from build123d import *

# Parameters (mm, degrees)
EXTRUDE_1_DEPTH           = 15.5
HOLE_WIZARD_M121_D        = 10.2
HOLE_WIZARD_M121_DEPTH    = 15.5
HOLE_WIZARD_M82_D         = 6.8
HOLE_WIZARD_M82_DEPTH     = 15.5
HOLE_WIZARD_8_0_8_1_D     = 8
HOLE_WIZARD_8_0_8_1_DEPTH = 15.5
SKETCH_9_W                = 8
SKETCH_9_H                = 8
SKETCH_9_H_2              = 5
SKETCH_9_W_2              = 5
EXTRUDE_2_DEPTH           = 2
FILLET_1_R                = 2


with BuildPart() as part:
    # Эскиз1 → Бобышка-Вытянуть1 (new body)
    with BuildSketch(Plane(origin=(0, 0, 0), x_dir=(1, 0, 0), z_dir=(0, 1, 0))):
        Polygon((0, 0), (0, 120), (60, 120), (120, 60), (120, 0), align=None)
    extrude(amount=EXTRUDE_1_DEPTH)

    # Отверстие обработанное метчиком M121
    with Locations(Plane(origin=(0, 15.5, 0), x_dir=(1, 0, 0), z_dir=(0, 1, 0))):
        with Locations((60, 60)):
            Hole(HOLE_WIZARD_M121_D / 2, depth=HOLE_WIZARD_M121_DEPTH)

    # Отверстие обработанное метчиком M82
    with Locations(Plane(origin=(0, 15.5, 0), x_dir=(1, 0, 0), z_dir=(0, 1, 0))):
        with Locations((58.180194847, 107.67766953), (107.67766953, 58.180194847), (58.180194847, 8.682720164), (8.682720164, 58.180194847)):
            Hole(HOLE_WIZARD_M82_D / 2, depth=HOLE_WIZARD_M82_DEPTH)

    # Диаметр отверстия Ø8.0 (8)1
    with Locations(Plane(origin=(0, 15.5, 0), x_dir=(1, 0, 0), z_dir=(0, 1, 0))):
        with Locations((20, 100), (20, 68), (20, 20), (68, 20), (100, 20)):
            Hole(HOLE_WIZARD_8_0_8_1_D / 2, depth=HOLE_WIZARD_8_0_8_1_DEPTH)

    # Эскиз9 → Бобышка-Вытянуть2 (add)
    with BuildSketch(Plane(origin=(0, 15.5, 0), x_dir=(1, 0, 0), z_dir=(0, 1, 0))):
        with Locations((20, 112)):
            Rectangle(SKETCH_9_W, SKETCH_9_H)
        with Locations((20, 80)):
            Rectangle(SKETCH_9_W, SKETCH_9_H)
        with Locations((20, 48.75)):
            Rectangle(SKETCH_9_W, SKETCH_9_H_2)
        with Locations((48.75, 20)):
            Rectangle(SKETCH_9_W_2, SKETCH_9_H)
        with Locations((80, 20)):
            Rectangle(SKETCH_9_W, SKETCH_9_H)
        with Locations((112, 20)):
            Rectangle(SKETCH_9_W, SKETCH_9_H)
    extrude(amount=EXTRUDE_2_DEPTH)

    # Скругление1
    fillet_1_edges = [part.edges().sort_by_distance(p)[0] for p in [
        (0, 7.75, 0),
        (0, 7.75, -120),
        (60, 7.75, -120),
        (120, 7.75, -60),
        (120, 7.75, 0),
    ]]
    fillet(fillet_1_edges, radius=FILLET_1_R)


solid = part.part
Model file for the job. Use its own axes, mm. Give positions to 0.01 mm unless a question says otherwise; leave off trailing zeros. Loops run counter-clockwise (first coordinate to the right, second up) from the corner with the lowest first, then second, coordinate; pieces in that order, holes last.
1) Saw through at A-A (z = -20). Write the cut outline in (x, y).
2) Pull direction X, two halves, no side cores. Call faces 1 (the flat face through (120, 8, -31)), 2 (the flat face through (112, 17.5, -20)), 3 (the cylindrical face through (102.95, 7.64, -22.7)): +X half, -X half, draft (parallel to the pull), parting line (faces both ways), or undercut.
3) Saw through at C-C (z = -102.5). Write the cut outline in (x, y), plus the area to 3 significant figures.
4) Saw through at B-B (x = 20). Write the cut outline in (y, z).
5) Wall check: line 1 (X direction, y = 8.25, z = -20); line 2 (Z direction, x = 20, y = 6.25); line 3 (X direction, y = 13.75, z = -59.5). Give the ranges that are in metal, low to high.
6) Saw through at D-D (y = 14). Count the separate pieces of the cut face and the enclosed holes in it, plus the area to 3 significant figures.
7) Flat gauge pins, fed straight in: pin 1 Ø4 at (x, z) = (107.68, -58.18) entering from +Y; pin 2 Ø2 at (x, z) = (56, -89) entering from -Y; pin 3 Ø1 at (x, y) = (19.5, 17) entering from +Z; pin 4 Ø0.6 at (y, z) = (16, -81.5) entering from +X. Where does each tip first touch, or does it go through?
Answer block:
1. outline: (0, 0) - (16, 0) - (16, 15.5) - (0, 15.5) - close; (24, 0) - (64, 0) - (64, 15.5) - (51.25, 15.5) - (51.25, 17.5) - (46.25, 17.5) - (46.25, 15.5) - (24, 15.5) - close; (72, 0) - (96, 0) - (96, 15.5) - (84, 15.5) - (84, 17.5) - (76, 17.5) - (76, 15.5) - (72, 15.5) - close; (104, 0) - (120, 0) - (120, 15.5) - (116, 15.5) - (116, 17.5) - (108, 17.5) - (108, 15.5) - (104, 15.5) - close
2. face 1: +X half
2. face 2: draft
2. face 3: undercut
3. outline: (0, 0) - (16.88, 0) - (16.88, 15.5) - (0, 15.5) - close; (23.12, 0) - (77.5, 0) - (77.5, 15.5) - (23.12, 15.5) - close
3. area: 1,100 mm2
4. outline: (0, -120) - (15.5, -120) - (15.5, -116) - (17.5, -116) - (17.5, -108) - (15.5, -108) - (15.5, -104) - (0, -104) - close; (0, -96) - (15.5, -96) - (15.5, -84) - (17.5, -84) - (17.5, -76) - (15.5, -76) - (15.5, -72) - (0, -72) - close; (0, -64) - (15.5, -64) - (15.5, -51.25) - (17.5, -51.25) - (17.5, -46.25) - (15.5, -46.25) - (15.5, -24) - (0, -24) - close; (0, -16) - (15.5, -16) - (15.5, 0) - (0, 0) - close
5. line 1: x = 0 to 16, 24 to 64, 72 to 96, 104 to 120
5. line 2: z = -120 to -104, -96 to -72, -64 to -24, -16 to 0
5. line 3: x = 0 to 5.55, 11.82 to 54.92, 65.08 to 104.54, 110.81 to 119.97
6. separate pieces: 1
6. enclosed holes: 10
6. area: 12,100 mm2
7. pin 1: passes through
7. pin 2: stops at y = 0
7. pin 3: stops at z = -46.25
7. pin 4: stops at x = 24
